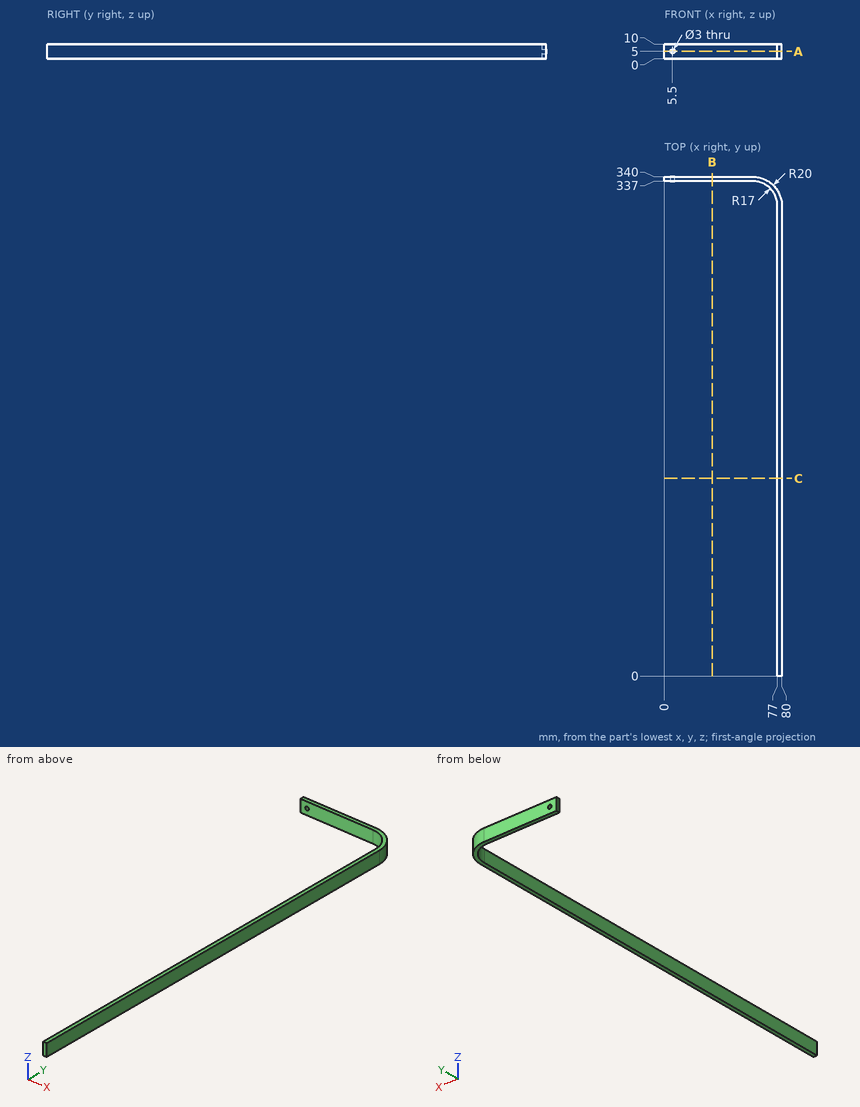
Design review of the part shown in the three views and the two pictorial views. Dimensions are in mm from the part's minimum x, y and z. Coordinates: 2 decimals unless noted, no trailing zeros. Order: outer loops, then holes, each group sorted by start corner. A loop starts at its lowest first (then second) coordinate and runs counter-clockwise, first axis right, second up.
1) Take a section at C-C, the plane y = 134.5. Give the boundary of the cut face in (x, z), and give its area (3 significant figures).
2) Take a section at B-B, the plane x = 32.5. Give the boundary of the cut face in (y, z), and give its area (3 significant figures).
3) Take a section at A-A, the plane z = 5. Give the boundary of the cut face in (x, y).
4) Wall thickness on line 1 along Z through (x, y) = (5.5, 339.45); line 2 along Y through (x, z) = (4, 4.5); line 3 along X through (y, z) = (284, 6): over which ranges is each line inside the solid? List them lowest first.
5) Clearance check with flat-ended pins moving along their axes: pin 1 (5 mm diameter, centred on y = 166, z = 7.5, fed in from -X); pin 2 (2.5 mm diameter, centred on x = 5.5, z = 5, fed in from +Y). State where each tip first meets the part, or that it passes through.
Returned:
1. outline: (77, 0) - (80, 0) - (80, 10) - (77, 10) - close
1. area: 30.0 mm2
2. outline: (337, 0) - (340, 0) - (340, 10) - (337, 10) - close
2. area: 30.0 mm2
3. outline: (0, 337) - (4, 337) - (4, 340) - (0, 340) - close; (7, 337) - (60, 337) arc R17 cw to (77, 320) - (77, 0) - (80, 0) - (80, 320) arc R20 ccw to (60, 340) - (7, 340) - close
4. line 1: z = 0 to 3.5, 6.5 to 10
4. line 2: y = 337 to 340
4. line 3: x = 77 to 80
5. pin 1: stops at x = 77
5. pin 2: passes through
